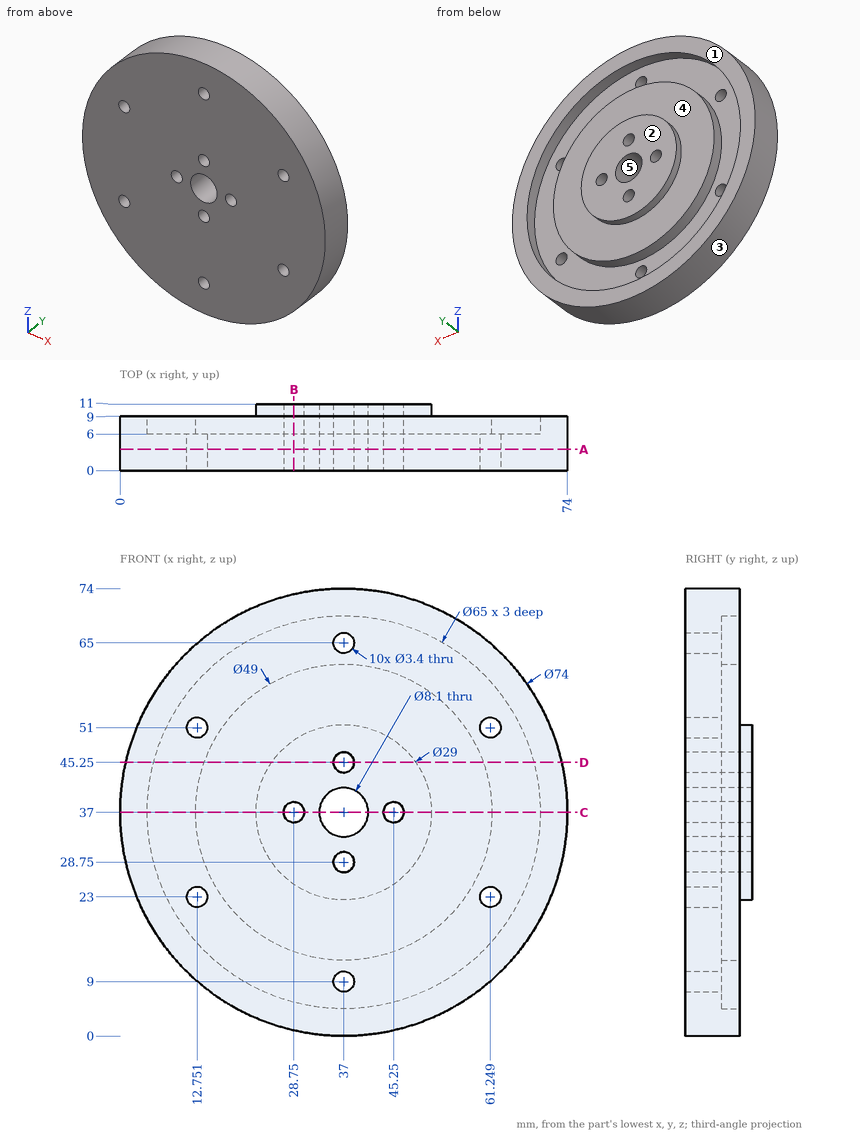
Could you check a few things on this drawing? It's one solid part, dimensions in mm from its lowest x, y, z. A direction names the side the tool comes from. Coordinates: 2 decimals unless noted, no trailing zeros. Loops run counter-clockwise (first coordinate to the right, second up) from the corner with the lowest first, then second, coordinate; pieces in that order, holes last.
1. We'd pull the mould along X, two halves only. Please class the marked faces 3, 4 and 5: released by +X, released by -X, zero draft, split by the parting line, or undercut.
2. For P1, Ø5.5, axis at x = 37, z = 9, coming from the +Y side; P2, Ø1, axis at y = 3, z = 59.5, coming from the -X side; P3, Ø1.5, axis at x = 14.5, y = 7.5, coming from the -Z side, each with a flat end and sliding along its axis, tell me the tip position at first contact or that it passes through.
3. I need wall thicknesses on L1, parallel to Z at x = 37, y = 5; L2, parallel to Z at x = 50, y = 6.75; L3, parallel to Z at x = 24.5, y = 7 (1 decimal). Which ranges of each line are inside material? Lowest first, please.
4. Imagine slicing it at A-A (y = 3.5). Give the number of separate pieces and of enclosed holes in the cut face, and give its area (3 significant figures).
5. Imagine slicing it at B-B (x = 28.75). Please give me the cut outline in (y, z) (1 decimal), and give its area (3 significant figures).
6. Imagine slicing it at C-C (z = 37). Please give me the cut outline in (x, y), and give its area (3 significant figures).
7. Imagine slicing it at D-D (z = 45.25). Please give me the cut outline in (x, y) (1 decimal).
8. For the marked faces 1 and 2, which set-ups out of +Z, -Z, +X, -X, +Y, -Y let a thin tool reach every point of the face, with its end or its side?
Computed values:
1. face 3: split by the parting line
1. face 4: zero draft
1. face 5: undercut
2. P1: stops at y = 6
2. P2: stops at x = 7.25
2. P3: stops at z = 7.07
3. L1: z = 0 to 7.3, 10.7 to 27.05, 30.45 to 32.95, 41.05 to 43.55, 46.95 to 63.3, 66.7 to 74
3. L2: z = 2.36 to 7.21, 16.23 to 57.77, 66.79 to 71.64
3. L3: z = 2.2 to 7, 15.9 to 58.1, 67 to 71.8
4. separate pieces: 1
4. enclosed holes: 11
4. area: 4,160 mm2
5. outline: (0, 0.9) - (9, 0.9) - (9, 5.6) - (6, 5.6) - (6, 13.9) - (9, 13.9) - (9, 25.1) - (11, 25.1) - (11, 35.3) - (0, 35.3) - close; (0, 38.7) - (11, 38.7) - (11, 48.9) - (9, 48.9) - (9, 60.1) - (6, 60.1) - (6, 68.4) - (9, 68.4) - (9, 73.1) - (0, 73.1) - close
5. area: 609 mm2
6. outline: (0, 0) - (27.05, 0) - (27.05, 11) - (22.5, 11) - (22.5, 9) - (12.5, 9) - (12.5, 6) - (4.5, 6) - (4.5, 9) - (0, 9) - close; (30.45, 0) - (32.95, 0) - (32.95, 11) - (30.45, 11) - close; (41.05, 0) - (43.55, 0) - (43.55, 11) - (41.05, 11) - close; (46.95, 0) - (74, 0) - (74, 9) - (69.5, 9) - (69.5, 6) - (61.5, 6) - (61.5, 9) - (51.5, 9) - (51.5, 11) - (46.95, 11) - close
6. area: 512 mm2
7. outline: (0.9, 0) - (35.3, 0) - (35.3, 11) - (25.1, 11) - (25.1, 9) - (13.9, 9) - (13.9, 6) - (5.6, 6) - (5.6, 9) - (0.9, 9) - close; (38.7, 0) - (73.1, 0) - (73.1, 9) - (68.4, 9) - (68.4, 6) - (60.1, 6) - (60.1, 9) - (48.9, 9) - (48.9, 11) - (38.7, 11) - close
8. face 1: +Y
8. face 2: +Z, -Z, +X, -X, +Y
